Verification items for this drawing (mm, ordinates from the low corner). Round coordinates to 2 decimals unless told otherwise and drop trailing zeros. Order: outer loops, then holes, each group sorted by start corner. A loop starts at its lowest first (then second) coordinate and runs counter-clockwise, first axis right, second up. Notation, with made-up numbers: (37, -20.75) -> (65, -20.75) arc R25 ccw to (65, 9.25) -> close; hole circle Ø11 at (40.5, 52.5). An arc over 180 degrees is marked (long way). Answer in a Markdown table with one row per item. Add a question column.
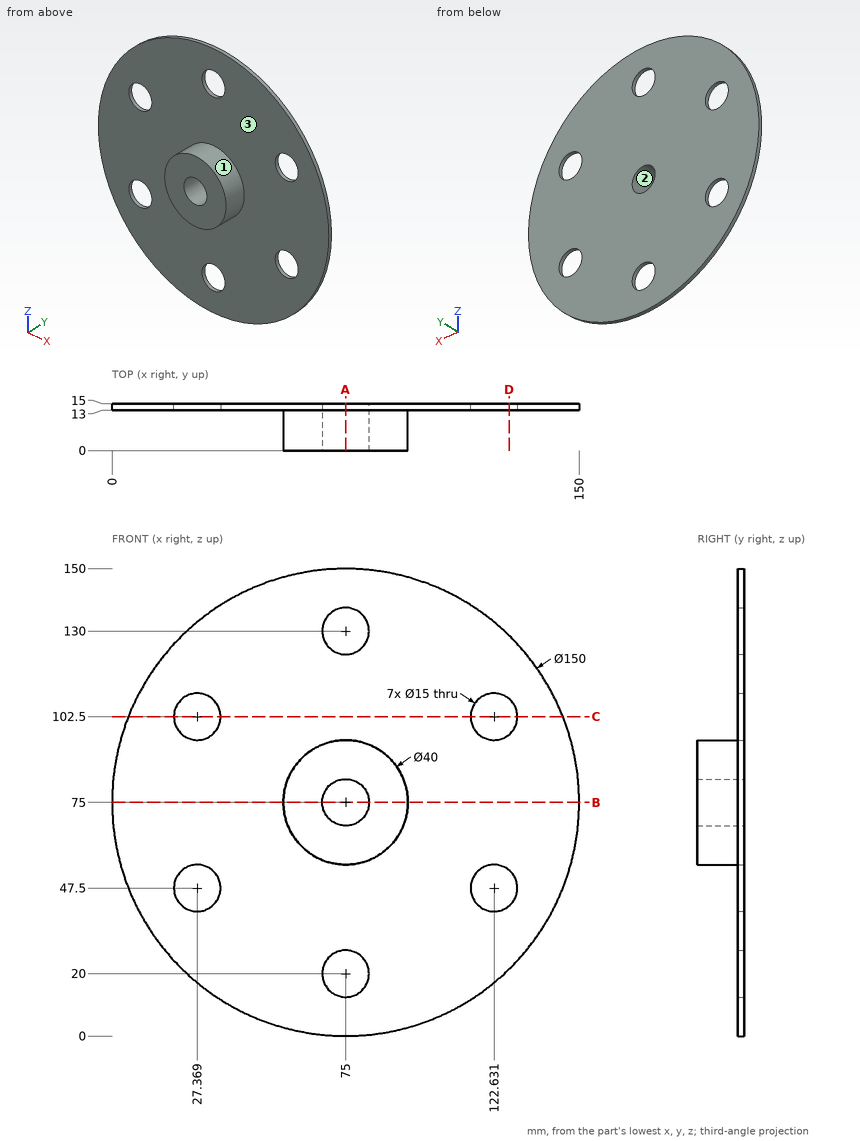
1) Cross-section at C-C, the plane z = 102.5. Record the boundary of the cut face in (x, y), and give its area (3 significant figures).
2) Cross-section at D-D, the plane x = 127.5. Record the boundary of the cut face in (y, z) (1 decimal).
3) Draft check along X on the marked faces 1, 2 and 3. Enter one of: +X half, -X half, draft (parallel to the pull), parting line (faces both ways), or undercut.
4) Thickness scan on L1, parallel to Z at x = 75, y = 14.15; L2, parallel to Z at x = 74.5, y = 1.5. Record the ranges inside material, lowest first. Write a range as [from, to].
5) Cross-section at B-B, the plane z = 75. Record the boundary of the cut face in (x, y), and give its area (3 significant figures).
6) Cross-section at A-A, the plane x = 75. Record the boundary of the cut face in (y, z).
7) Depth check by flat-ended pin: P1, Ø8, axis at y = 10.5, z = 26, coming from the -X side; P2, Ø6, axis at x = 100.5, y = 12.5, coming from the +Z side; P3, Ø12, axis at x = 126, z = 88.5, coming from the -Y side. Enter the tip coordinate at first touch or a pass-through.
Results below:
| question | item | result |
|---|---|---|
| 1 | outline | (5.22, 13) -> (19.87, 13) -> (19.87, 15) -> (5.22, 15) -> close; (34.87, 13) -> (115.13, 13) -> (115.13, 15) -> (34.87, 15) -> close; (130.13, 13) -> (144.78, 13) -> (144.78, 15) -> (130.13, 15) -> close |
| 1 | area | 219 mm² |
| 2 | outline | (13, 21.4) -> (15, 21.4) -> (15, 41.8) -> (13, 41.8) -> close; (13, 53.2) -> (15, 53.2) -> (15, 96.8) -> (13, 96.8) -> close; (13, 108.2) -> (15, 108.2) -> (15, 128.6) -> (13, 128.6) -> close |
| 3 | face 1 | parting line |
| 3 | face 2 | undercut |
| 3 | face 3 | draft |
| 4 | L1 | [0, 12.5], [27.5, 67.5], [82.5, 122.5], [137.5, 150] |
| 4 | L2 | [55.01, 67.52], [82.48, 94.99] |
| 5 | outline | (0, 13) -> (55, 13) -> (55, 0) -> (67.5, 0) -> (67.5, 15) -> (0, 15) -> close; (82.5, 0) -> (95, 0) -> (95, 13) -> (150, 13) -> (150, 15) -> (82.5, 15) -> close |
| 5 | area | 595 mm² |
| 6 | outline | (0, 55) -> (13, 55) -> (13, 27.5) -> (15, 27.5) -> (15, 67.5) -> (0, 67.5) -> close; (0, 82.5) -> (15, 82.5) -> (15, 122.5) -> (13, 122.5) -> (13, 95) -> (0, 95) -> close; (13, 0) -> (15, 0) -> (15, 12.5) -> (13, 12.5) -> close; (13, 137.5) -> (15, 137.5) -> (15, 150) -> (13, 150) -> close |
| 7 | P1 | x = 15.67 |
| 7 | P2 | z = 146.53 |
| 7 | P3 | y = 13 |
